```python
from build123d import *

# Parameters (mm, degrees)
SALIENTE_EXTRUIR1_DEPTH = 4
CROQUIS4_W              = 113.4
CROQUIS4_H              = 2
CORTAR_EXTRUIR1_DEPTH   = 10
REDONDEO1_R             = 2
CROQUIS5_W              = 115.9
CROQUIS5_H              = 31.071267716
CORTAR_EXTRUIR2_DEPTH   = 2


with BuildPart() as part:
    # Croquis1 → Saliente-Extruir1 (new body)
    with BuildSketch(Plane(origin=(0, 0, 0), x_dir=(1, 0, 0), z_dir=(0, 1, 0))):
        Polygon((-65.583943666, 30.054443615), (49.816056334, 30.054443615), (49.816056334, 33.054443615), (51.916056334, 33.054443615), (51.916056334, 30.054443615), (51.916056334, -4.445556385), (-67.683943666, -4.445556385), (-67.683943666, 30.054443615), (-67.683943666, 33.054443615), (-65.583943666, 33.054443615), align=None)
    extrude(amount=SALIENTE_EXTRUIR1_DEPTH)

    # Croquis4 → Cortar-Extruir1 (cut)
    with BuildSketch(Plane(origin=(0, 4, 0), x_dir=(1, 0, 0), z_dir=(0, 1, 0))):
        with Locations((-7.883943666, 29.054443615)):
            Rectangle(CROQUIS4_W, CROQUIS4_H)
        with BuildLine():
            Line((49.816056334, 26.054443615), (49.816056334, 30.054443615))
            Line((49.816056334, 30.054443615), (48.816056334, 30.054443615))
            Line((48.816056334, 30.054443615), (48.816056334, 28.054443615))
            Line((48.816056334, 28.054443615), (48.816056334, 26.054443615))
            ThreePointArc((48.816056334, 26.054443615), (49.316056334, 25.554443615), (49.816056334, 26.054443615))
        make_face()
        with BuildLine():
            Line((-64.583943666, 28.054443615), (-64.583943666, 30.054443615))
            Line((-64.583943666, 30.054443615), (-65.583943666, 30.054443615))
            Line((-65.583943666, 30.054443615), (-65.583943666, 26.054443615))
            ThreePointArc((-65.583943666, 26.054443615), (-65.083943666, 25.554443615), (-64.583943666, 26.054443615))
            Line((-64.583943666, 26.054443615), (-64.583943666, 28.054443615))
        make_face()
    extrude(amount=-CORTAR_EXTRUIR1_DEPTH, mode=Mode.SUBTRACT)

    # Redondeo1
    redondeo1_edges = [part.edges().sort_by_distance(p)[0] for p in [
        (-66.633943666, 0, -33.054443615),
        (-66.633943666, 4, -33.054443615),
        (50.866056334, 0, -33.054443615),
        (50.866056334, 4, -33.054443615),
    ]]
    fillet(redondeo1_edges, radius=REDONDEO1_R - 0.0001)  # a hair under: the kernel refuses the full size

    # Croquis3 → Revolución1 (revolve)
    with BuildSketch(Plane(origin=(-65.583943666, 0, 0), x_dir=(0, 0, -1), z_dir=(1, 0, 0))):
        with BuildLine():
            Line((32.054443615, 2), (30.054443615, 2))
            ThreePointArc((30.054443615, 2), (31.054443615, 1), (32.054443615, 2))
        make_face()
    revolve(axis=Axis((-65.583943666, 2, -32.054443615), (0, 0, 1)))

    # Croquis2 → Revolución2 (revolve)
    with BuildSketch(Plane.ZY.offset(-49.816056334)):
        with BuildLine():
            Line((-32.054443615, 2), (-30.054443615, 2))
            ThreePointArc((-30.054443615, 2), (-31.054443615, 1), (-32.054443615, 2))
        make_face()
    revolve(axis=Axis((49.816056334, 2, -32.054443615), (0, 0, 1)))

    # Croquis5 → Cortar-Extruir2 (cut)
    with BuildSketch(Plane(origin=(0, 4, 0), x_dir=(1, 0, 0), z_dir=(0, 1, 0))):
        with Locations((-7.633943666, 14.090077473)):
            Rectangle(CROQUIS5_W, CROQUIS5_H)
    extrude(amount=-CORTAR_EXTRUIR2_DEPTH, mode=Mode.SUBTRACT)


solid = part.part
```
Could you check a few things on this model? Use its own coordinates, in mm. A direction names the side the tool comes from. Round coordinates to 2 decimals unless told otherwise and drop trailing zeros. Loops run counter-clockwise (first coordinate to the right, second up) from the corner with the lowest first, then second, coordinate; pieces in that order, holes last. Notation, with made-up numbers: M 78.5,77.25 L 82.5,77.25 A25 cw 82.5,114.25 Z; hole C 34.25,-38.75 d11. An arc over 180 degrees is marked long. Write item = value, one per line.
1. I want a section at B-B, the plane x = 22. Write out the boundary of the cut face in (y, z), and give its area (3 significant figures).
Results below:
outline = M 0,-28.05 L 2,-28.05 L 2,1.45 L 4,1.45 L 4,4.45 L 0,4.45 Z
area = 71.0 mm²
2. Will these pins go through, and if not, where does the flat tip stop? P1, Ø6, axis at x = -50, z = -19, coming from the +Y side; P2, Ø1.6, axis at x = -13, y = 1, coming from the -Z side; P3, Ø1.5, axis at x = -51, y = 3.5, coming from the -Z side.
Results below:
P1 = 2
P2 = -28.05
P3 = 1.45
3. I want a section at A-A, the plane z = -5.5. Write out the boundary of the cut face in (x, y).
Results below:
outline = M -67.68,0 L 51.92,0 L 51.92,4 L 50.32,4 L 50.32,2 L -65.58,2 L -65.58,4 L -67.68,4 Z
4. Thinking about a two-plate mould opening in X: for faces 4 (the face through (-67.684, 2, -15)), 5 (the face through (-66.62, 0.57, -32.45)), 6 (the face through (50.316, 3, -14)), 7 (the face through (51.916, 2, -14)), which applies, +X half, -X half, draft (parallel to the pull), parting line (faces both ways), or undercut?
Results below:
face_4 = -X half
face_5 = draft
face_6 = undercut
face_7 = +X half
5. Which directions (+Z, -Z, +X, -X, +Y, -Y) give clear straight access to the entire face, cutting with the end or side of a thin tool? Please do faces 1 (the face through (50.88, 0.57, -32.45)), 2 (the face through (-9, 1, -28.054)), 3 (the face through (49.816, 1.5, -29.5)).
Results below:
face_1 = -Z, +X, -X, -Y
face_2 = -Z, +Y, -Y
face_3 = none
6. I need wall thicknesses on probe 1 along X at (y, z) = (2.1, -25); probe 2 along X at (y, z) = (0.7, -30.5); probe 3 along Z at (x, y) = (12, 2.5). Which ranges of each line are inside material? Lowest first, please.
Results below:
probe_1 = -67.68 to -65.58, 50.32 to 51.92
probe_2 = -67.68 to -65.58, 49.82 to 51.92
probe_3 = 1.45 to 4.45
